Build history of the part. All positions in model axes, mm. A direction names the side the tool comes from. Give positions to 0.01 mm unless a question says otherwise; leave off trailing zeros. Write each loop counter-clockwise with the first axis right and the second up, starting at its lowest first coordinate (ties: lowest second). Pieces come first, ordered by that corner, then holes. Notation, with made-up numbers: M -19.5,14.25 L -5.5,14.25 A5 ccw -5.5,20.25 Z; hole C 8.5,18.25 d6. An arc over 180 degrees is marked long. Return JSON: item names as keys, results as strings. Group by question number.
Q1. Band-saw the part on B-B, the plane z = 2.3. Count the separate pieces of the cut face and the enclosed holes in it, then the cut area to 3 significant figures.
Q2. Wall check: probe 1 along X at (y, z) = (15, 1.6); probe 2 along Y at (x, z) = (5.25, 0.35); probe 3 along Y at (x, z) = (3.75, 0.55). Give the ranges that are in metal, low to high.
Q3. Tool access for faces 4 (the flat face through (5, 0, 1)), 5 (the flat face through (-7, 1, 0)), 6 (the cylindrical face through (6.58, 44.883, 2.014)): list every direction of +Z, -Z, +X, -X, +Y, -Y with a clear straight run to the whole face (end or side of a thin tool).
Q4. Pull direction X, two halves, no side cores. Call faces 1 (the flat face through (-7, 1, 3)), 2 (the cylindrical face through (0, -52, 1)), 3 (the cylindrical face through (-6.258, 48.564, 2.014)): +X half, -X half, draft (parallel to the pull), parting line (faces both ways), or undercut.
Q5. Band-saw the part on A-A, the plane y = 19. Give the cut face in (x, z).
Q6. Flat gauge pins, fed straight in: pin 1 Ø1.2 at (x, y) = (-6.5, 46) entering from +Z; pin 2 Ø1 at (x, z) = (6.5, 1) entering from -Y. Where does each tip first touch, or does it go through?
from build123d import *

# Parameters (mm, degrees)
BOSS_EXTRUDE1_DEPTH = 3
SKETCH3_R           = 4.25
SKETCH3_R_2         = 1.1
CUT_EXTRUDE3_DEPTH  = 3
SKETCH3_6_R         = 2
CUT_EXTRUDE4_DEPTH  = 2
CIRPATTERN3_COUNT   = 4
SKETCH2_R           = 3.05
SKETCH2_R_2         = 1
CUT_EXTRUDE5_DEPTH  = 3
SKETCH2_5_R         = 2
CUT_EXTRUDE6_DEPTH  = 2
CIRPATTERN4_COUNT   = 4
FILLET1_R           = 3


with BuildPart() as part:
    # Sketch1 → Boss-Extrude1 (new body)
    with BuildSketch(Plane.XY):
        with BuildLine():
            ThreePointArc((11, 41), (0, 52), (-11, 41))
            Line((-11, 41), (-11, -41))
            ThreePointArc((-11, -41), (0, -52), (11, -41))
            Line((11, -41), (11, 41))
        make_face()
        with BuildLine():
            ThreePointArc((0, 30), (2.571230378, 30.304731217), (5, 31.202041029))
            Line((5, 31.202041029), (5, -31.202041029))
            ThreePointArc((5, -31.202041029), (2.571230378, -30.304731217), (0, -30))
            ThreePointArc((0, -30), (-2.571230378, -30.304731217), (-5, -31.202041029))
            Line((-5, -31.202041029), (-5, 31.202041029))
            ThreePointArc((-5, 31.202041029), (-2.571230378, 30.304731217), (0, 30))
        make_face(mode=Mode.SUBTRACT)
    extrude(amount=BOSS_EXTRUDE1_DEPTH)

    # Sketch3 → Cut-Extrude3 (cut)
    with BuildSketch(Plane.XY.offset(3)):
        with Locations((0, -41)):
            Circle(SKETCH3_R)
        with Locations((5.656854249, -35.343145751)):
            Circle(SKETCH3_R_2)
    cut_extrude3 = extrude(amount=-CUT_EXTRUDE3_DEPTH, mode=Mode.SUBTRACT)

    # Sketch3<6> → Cut-Extrude4 (cut)
    with BuildSketch(Plane.XY.offset(3)):
        with Locations((5.656854249, -35.343145751)):
            Circle(SKETCH3_6_R)
    cut_extrude4 = extrude(amount=-CUT_EXTRUDE4_DEPTH, mode=Mode.SUBTRACT)

    # CirPattern3: Cut-Extrude3, Cut-Extrude4 ×4 about axis
    cirpattern3_axis = Axis((0, -41, 0), (0, 0, 1))
    add([cut_extrude3.rotate(cirpattern3_axis, i * 360 / CIRPATTERN3_COUNT) for i in range(1, CIRPATTERN3_COUNT)], mode=Mode.SUBTRACT)
    add([cut_extrude4.rotate(cirpattern3_axis, i * 360 / CIRPATTERN3_COUNT) for i in range(1, CIRPATTERN3_COUNT)], mode=Mode.SUBTRACT)

    # Sketch2 → Cut-Extrude5 (cut)
    with BuildSketch(Plane.XY.offset(3)):
        with Locations((0, 41)):
            Circle(SKETCH2_R)
        with Locations((5.656854249, 46.656854249)):
            Circle(SKETCH2_R_2)
    cut_extrude5 = extrude(amount=-CUT_EXTRUDE5_DEPTH, mode=Mode.SUBTRACT)

    # Sketch2<5> → Cut-Extrude6 (cut)
    with BuildSketch(Plane.XY.offset(3)):
        with Locations((5.656854249, 46.656854249)):
            Circle(SKETCH2_5_R)
    cut_extrude6 = extrude(amount=-CUT_EXTRUDE6_DEPTH, mode=Mode.SUBTRACT)

    # CirPattern4: Cut-Extrude5, Cut-Extrude6 ×4 about axis
    cirpattern4_axis = Axis((0, 41, 0), (0, 0, 1))
    add([cut_extrude5.rotate(cirpattern4_axis, i * 360 / CIRPATTERN4_COUNT) for i in range(1, CIRPATTERN4_COUNT)], mode=Mode.SUBTRACT)
    add([cut_extrude6.rotate(cirpattern4_axis, i * 360 / CIRPATTERN4_COUNT) for i in range(1, CIRPATTERN4_COUNT)], mode=Mode.SUBTRACT)

    # Fillet1
    fillet1_edges = [part.edges().sort_by_distance(p)[0] for p in [
        (5, 31.202041029, 1.5),
        (-5, 31.202041029, 1.5),
        (-5, -31.202041029, 1.5),
        (5, -31.202041029, 1.5),
    ]]
    fillet(fillet1_edges, radius=FILLET1_R)


solid = part.part
From the geometry:
{
 "1": {"separate pieces": "1", "enclosed holes": "11", "area": "1,400 mm^2"},
 "2": {"probe 1": "x = -11 to -5, 5 to 11", "probe 2": "y = -50.67 to -47.68, -45.63 to -36.37, -34.32 to 34.43, 36.26 to 45.74, 47.57 to 50.67", "probe 3": "y = -51.34 to -43, -39 to -29.58, 29.58 to 51.34"},
 "3": {"face 4": "+Z, -Z", "face 5": "-Z, +X, -X, +Y, -Y", "face 6": "+Z"},
 "4": {"face 1": "draft", "face 2": "parting line", "face 3": "undercut"},
 "5": {"outline": "M -11,0 L -5,0 L -5,3 L -11,3 Z; M 5,0 L 11,0 L 11,3 L 5,3 Z"},
 "6": {"pin 1": "stops at z = 1", "pin 2": "stops at y = -50.22"}
}
